Source: CAD feature listing. Evaluate the final solid. Frame: model axes, mm. Give positions to 0.01 mm unless a question says otherwise; leave off trailing zeros. Order: outer loops, then holes, each group sorted by start corner. A loop starts at its lowest first (then second) coordinate and runs counter-clockwise, first axis right, second up. Notation, with made-up numbers: (79.5, 3.25) - (104.5, 3.25) arc R31 ccw to (104.5, 35.25) - close; hole circle Ø9 at (-12, 15.5). An arc over 180 degrees is marked (long way). Answer as CSV lines item,"result".
```python
from build123d import *

# Parameters (mm, degrees)
SKETCH2_R           = 6.35
BOSS_EXTRUDE1_DEPTH = 5.08


with BuildPart() as part:
    # Sketch2 → Boss-Extrude1 (new body)
    with BuildSketch(Plane(origin=(0, 0, 0), x_dir=(1, 0, 0), z_dir=(0, 0, -1))):
        with BuildLine():
            Line((-249.9, -70.6), (-249.9, 2.7))
            ThreePointArc((-249.9, 2.7), (-246.971067812, 9.771067812), (-239.9, 12.7))
            Line((-239.9, 12.7), (0, 12.7))
            ThreePointArc((0, 12.7), (12.7, 0), (0, -12.7))
            Line((0, -12.7), (-224.5, -12.7))
            Line((-224.5, -12.7), (-224.5, -70.6))
            ThreePointArc((-224.5, -70.6), (-237.2, -83.3), (-249.9, -70.6))
        make_face()
        with Locations(Location((0, 0, 0), (0, 0, 180))):
            Circle(SKETCH2_R, mode=Mode.SUBTRACT)
        with Locations((-237.2, -70.6)):
            Circle(SKETCH2_R, mode=Mode.SUBTRACT)
    extrude(amount=BOSS_EXTRUDE1_DEPTH)


solid = part.part
```
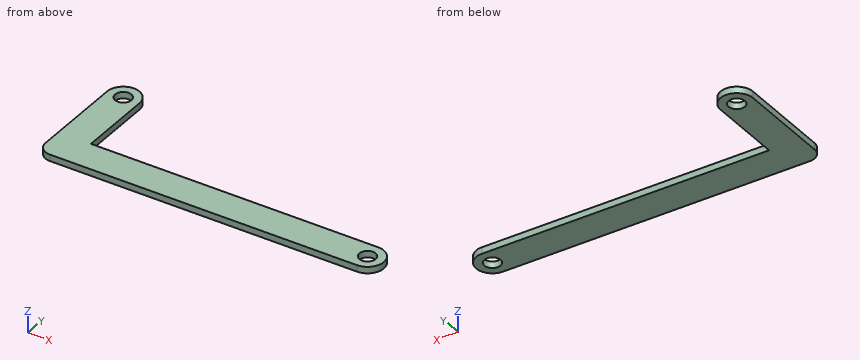
(1) Cut plane A-A (x = -237.2). Return loops of the section in (y, z).
Completed:
outline,"(-12.7, -5.08) - (64.25, -5.08) - (64.25, 0) - (-12.7, 0) - close; (76.95, -5.08) - (83.3, -5.08) - (83.3, 0) - (76.95, 0) - close"
(2) Cut plane B-B (z = -2.1). Return loops of the section in (x, y).
Completed:
outline,"(-249.9, -2.7) arc R10 ccw to (-239.9, -12.7) - (0, -12.7) arc R12.7 ccw to (0, 12.7) - (-224.5, 12.7) - (-224.5, 70.6) arc R12.7 ccw to (-249.9, 70.6) - close; hole circle Ø12.7 at (-237.2, 70.6); hole circle Ø12.7 at (0, 0)"
(3) Cut plane D-D (y = 39.5). Return loops of the section in (x, z).
Completed:
outline,"(-249.9, -5.08) - (-224.5, -5.08) - (-224.5, 0) - (-249.9, 0) - close"
(4) Ray query, line 1 (X direction, y = 70.6, z = -1.65); line 2 (Y direction, x = -237.2, z = -3.6); line 3 (Y direction, x = -217.5, z = -1.85). Return the intervals inside material, ascending. Write a range as from..to.
Completed:
line 1,"-249.9..-243.55, -230.85..-224.5"
line 2,"-12.7..64.25, 76.95..83.3"
line 3,"-12.7..12.7"
(5) Cut plane C-C (y = 0). Return loops of the section in (x, z), then the cut area to 3 significant figures.
Completed:
outline,"(-249.9, -5.08) - (-6.35, -5.08) - (-6.35, 0) - (-249.9, 0) - close; (6.35, -5.08) - (12.7, -5.08) - (12.7, 0) - (6.35, 0) - close"
area,"1,270 mm²"
